Answer from the drawing. Dimensions are ordinates in mm from the lowest x, y and z of the part. Give positions to 0.01 mm unless a question says otherwise; leave off trailing zeros. Loops run counter-clockwise (first coordinate to the right, second up) from the corner with the lowest first, then second, coordinate; pieces in that order, holes last. Notation, with made-up numbers: (26, 71) - (81, 71) arc R32 ccw to (81, 98) - close; hole circle Ø7 at (-17, 27.25). An arc over 180 degrees is marked (long way). One line per question, with ' | ' between items. Start each with the question number.
1. Each of these flat-tipped pins is pushed along its axis until it touches: pin 1 (0.5 mm diameter, centred on y = 3, z = 2.5, fed in from -X); pin 2 (1.1 mm diameter, centred on x = 11.5, y = 1.5, fed in from -Z). Where does it stop, or does it pass through?
2. Section C-C (z = 4) is taken. Determine the outline of the cut face in (x, y).
3. For a pull along X with two mould halves and no side action, classify the marked faces 1, 2 and 3 as released by +X, released by -X, zero draft, split by the parting line, or undercut.
4. Find the intervals of material crossed by line 1 (Y direction, x = 6, z = 9); line 2 (Z direction, x = 1.75, y = 3.9); line 3 (X direction, y = 2.35, z = 6.5), in increasing order.
5. Section B-B (y = 4.4) is taken. Determine the outline of the cut face in (x, z).
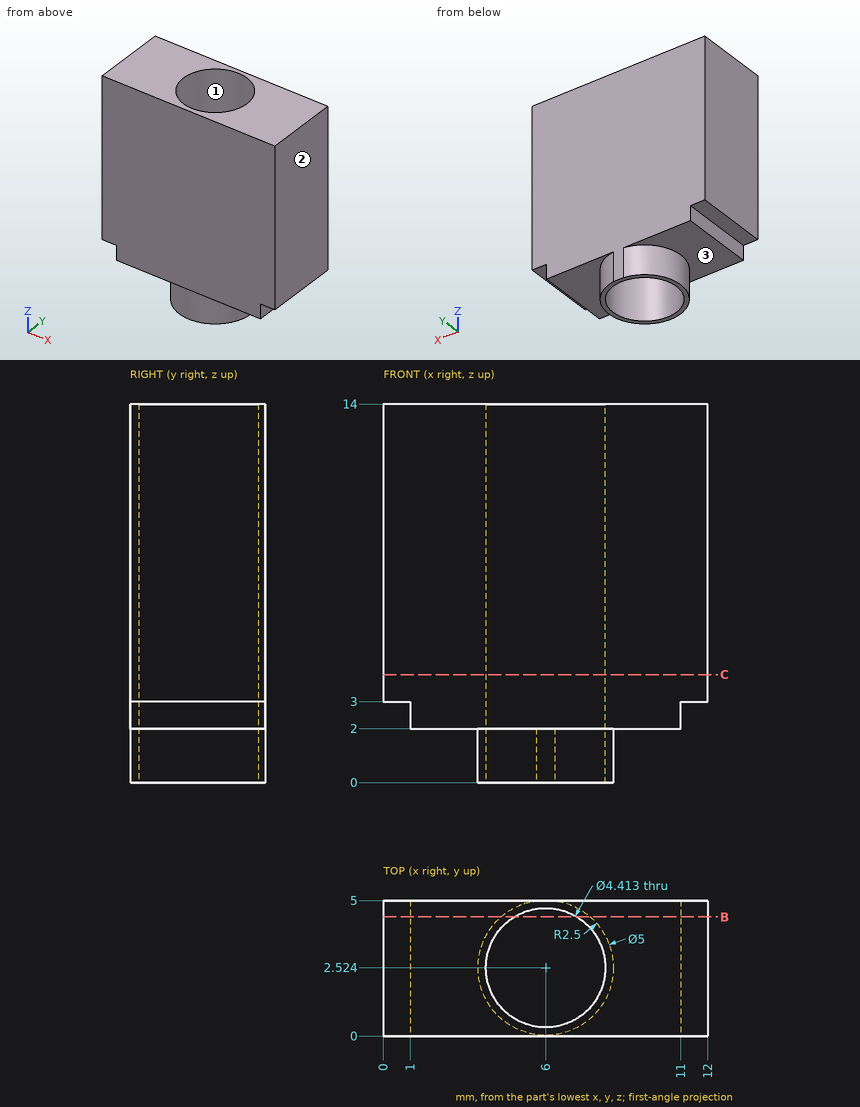
Conclusion:
1) pin 1: x = 1 | pin 2: z = 2
2) outline: (0, 0) - (12, 0) - (12, 5) - (0, 5) - close; hole circle Ø4.41 at (6, 2.52)
3) face 1: undercut | face 2: released by +X | face 3: zero draft
4) line 1: 0 to 0.32, 4.73 to 5 | line 2: 2 to 14 | line 3: 0 to 3.8, 8.2 to 12
5) outline: (0, 3) - (1, 3) - (1, 2) - (4.35, 2) - (4.35, 0) - (4.84, 0) - (4.84, 14) - (0, 14) - close; (7.16, 0) - (7.65, 0) - (7.65, 2) - (11, 2) - (11, 3) - (12, 3) - (12, 14) - (7.16, 14) - close
